Can you work these out from the drawing? Everything is in mm from the part's minimum corner. A direction names the side the tool comes from. Round coordinates to 2 decimals unless told otherwise and drop trailing zeros. Write each loop counter-clockwise with the first axis right and the second up, starting at its lowest first coordinate (ties: lowest second). Pieces come first, ordered by that corner, then holes. Notation, with made-up numbers: (-16, 64.5) - (13, 64.5) arc R9 ccw to (13, 79.5) - close; hole circle Ø10 at (37, -27). An arc over 180 degrees is marked (long way). One line per item, written item: value. Start each with the question number.
(1) I want a section at D-D on y = 12.5. List the corners of the cut face in (x, z) for me.
(2) I want a section at B-B on x = 45. List the corners of the cut face in (y, z) for me.
(3) I'm going to push flat-ended pins straight in: pin 1 Ø1.5 at (x, z) = (36, 66) entering from +Y; pin 2 Ø4 at (y, z) = (2, 71.5) entering from -X; pin 3 Ø1.5 at (x, y) = (78, 13.5) entering from -Z. Where does each tip first touch, or does it pass through?
(4) I want a section at C-C on x = 32. List the corners of the cut face in (y, z) for me.
(5) Thinking about a two-plate mould opening in Z: for the marked faces 1, 2 and 3, which applies, +Z half, -Z half, draft (parallel to the pull), parting line (faces both ways), or undercut?
(6) On a 3-axis mill with a long thin cutter (end or side, diameter ignored), from which of +Z, -Z, +X, -X, +Y, -Y can I reach the whole of each face in a straight line? I mean the marked faces 4 and 5. Say none if no direction works.
(7) If I drill on L1, parallel to X at y = 1.4, z = 45; L2, parallel to X at y = 10, z = 45; L3, parallel to X at y = 13.25, z = 65, over which ranges is the centre line in solid material (lowest first)? Write a range as from..to.
(8) I want a section at A-A on z = 45. List the corners of the cut face in (x, y) for me, plus the area to 3 significant figures.
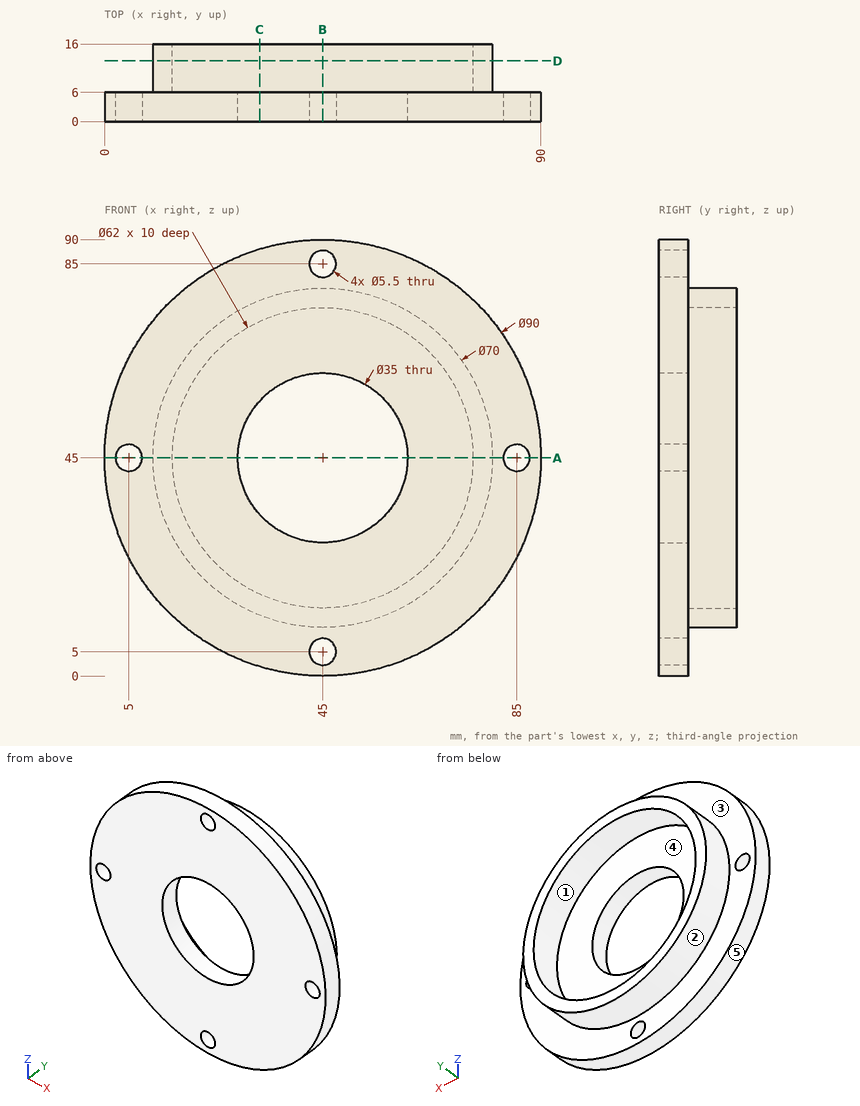
Established:
1. outline: circle Ø70 at (45, 45); hole circle Ø62 at (45, 45)
2. outline: (0, 0) - (6, 0) - (6, 2.25) - (0, 2.25) - close; (0, 7.75) - (6, 7.75) - (6, 10) - (16, 10) - (16, 14) - (6, 14) - (6, 27.5) - (0, 27.5) - close; (0, 62.5) - (6, 62.5) - (6, 76) - (16, 76) - (16, 80) - (6, 80) - (6, 82.25) - (0, 82.25) - close; (0, 87.75) - (6, 87.75) - (6, 90) - (0, 90) - close
3. pin 1: y = 6
3. pin 2: x = 7.25
3. pin 3: z = 31.4
4. outline: (0, 1.92) - (6, 1.92) - (6, 12.5) - (16, 12.5) - (16, 16.86) - (6, 16.86) - (6, 33.28) - (0, 33.28) - close; (0, 56.72) - (6, 56.72) - (6, 73.14) - (16, 73.14) - (16, 77.5) - (6, 77.5) - (6, 88.08) - (0, 88.08) - close
5. face 1: undercut
5. face 2: parting line
5. face 3: draft
6. face 4: +Y
6. face 5: +Y, -Y
7. L1: 0..2.25, 7.75..27.5, 62.5..82.25, 87.75..90
7. L2: 10..14, 76..80
7. L3: 16.28..21.31, 68.69..73.72
8. outline: (0, 0) - (2.25, 0) - (2.25, 6) - (0, 6) - close; (7.75, 0) - (27.5, 0) - (27.5, 6) - (14, 6) - (14, 16) - (10, 16) - (10, 6) - (7.75, 6) - close; (62.5, 0) - (82.25, 0) - (82.25, 6) - (80, 6) - (80, 16) - (76, 16) - (76, 6) - (62.5, 6) - close; (87.75, 0) - (90, 0) - (90, 6) - (87.75, 6) - close
8. area: 344 mm2
